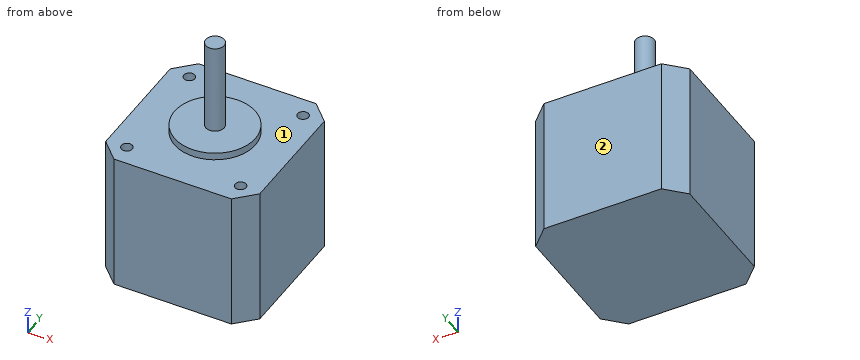
```python
from build123d import *

# Parameters (mm, degrees)
F0_W     = 42
F0_H     = 42
F1_DEPTH = 38
F2_SIZE  = 5
F3_R     = 11
F4_DEPTH = 2
F5_R     = 2.5
F6_DEPTH = 25
F7_R     = 1.5
F8_DEPTH = 25


with BuildPart() as f1:
    # F0 (on Top) → F1 (new body)
    with BuildSketch(Plane.XY):
        with Locations((21, 21)):
            Rectangle(F0_W, F0_H)
    extrude(amount=F1_DEPTH)

    # F2
    f2_edges = [f1.edges().sort_by_distance(p)[0] for p in [
        (0, 0, 19),
        (0, 42, 19),
        (42, 0, 19),
        (42, 42, 19),
    ]]
    chamfer(f2_edges, length=F2_SIZE)

    # F3 (on face) → F4 (join)
    with BuildSketch(Plane.XY.offset(38)):
        with Locations((21, 21)):
            Circle(F3_R)
    extrude(amount=F4_DEPTH)

    # F5 (on face) → F6 (join)
    with BuildSketch(Plane.XY.offset(40)):
        with Locations((21, 21)):
            Circle(F5_R)
    extrude(amount=F6_DEPTH)

    # F7 (on face) → F8 (cut)
    with BuildSketch(Plane.XY.offset(38)):
        with Locations((5.5, 36.5)):
            Circle(F7_R)
        with Locations((5.5, 5.5)):
            Circle(F7_R)
        with Locations((36.5, 36.5)):
            Circle(F7_R)
        with Locations((36.5, 5.5)):
            Circle(F7_R)
    extrude(amount=-F8_DEPTH, mode=Mode.SUBTRACT)


solid = f1.part
```
Geometry check sheet. Reference: the model listing, model coordinates, mm. Face numbers are marked on the shaded views. A direction names the side the tool comes from. Round coordinates to 2 decimals unless told otherwise and drop trailing zeros. Order: outer loops, then holes, each group sorted by start corner. A loop starts at its lowest first (then second) coordinate and runs counter-clockwise, first axis right, second up. Notation, with made-up numbers: (35.25, -36) - (84.25, -36) arc R20 ccw to (84.25, -10) - close; hole circle Ø7 at (44, 67). An arc over 180 degrees is marked (long way). Use a Markdown table: item, result. Add a question column.
1) Thickness scan on line 1 along Y through (x, z) = (36.5, 24); line 2 along X through (y, z) = (5, 26); line 3 along Z through (x, y) = (30, 32). Record the ranges inside material, lowest first.
2) Section check C-C (z = 26.5). Record the cut outline in (x, y).
3) Gauge pin test, flat ends, axial feed: P1, Ø12.5, axis at x = 18, y = 19.5, coming from the +Z side; P2, Ø0.9, axis at x = 36.5, y = 36, coming from the +Z side; P3, Ø12, axis at y = 10, z = 53.5, coming from the -X side; P4, Ø3.5, axis at x = 36.5, y = 36.5, coming from the +Z side. Record the tip position at first contact, or that the pin passes through.
4) Section check A-A (z = 11.5). Record the cut outline in (x, y).
5) Section check D-D (x = 16.5). Record the cut outline in (y, z), then the cut area to 3 significant figures.
6) Set-up check for the marked faces 1 and 2: record each of +Z, -Z, +X, -X, +Y, -Y from which the full face is reachable in a straight line by a thin tool's end or side.
7) Section check B-B (y = 21). Record the cut outline in (x, z), then the cut area to 4 significant figures.
Established:
| question | item | result |
|---|---|---|
| 1 | line 1 | 0 to 4, 7 to 35, 38 to 42 |
| 1 | line 2 | 0 to 4.09, 6.91 to 35.09, 37.91 to 42 |
| 1 | line 3 | 0 to 38 |
| 2 | outline | (0, 5) - (5, 0) - (37, 0) - (42, 5) - (42, 37) - (37, 42) - (5, 42) - (0, 37) - close; hole circle Ø3 at (5.5, 5.5); hole circle Ø3 at (5.5, 36.5); hole circle Ø3 at (36.5, 5.5); hole circle Ø3 at (36.5, 36.5) |
| 3 | P1 | z = 65 |
| 3 | P2 | z = 13 |
| 3 | P3 | through |
| 3 | P4 | z = 38 |
| 4 | outline | (0, 5) - (5, 0) - (37, 0) - (42, 5) - (42, 37) - (37, 42) - (5, 42) - (0, 37) - close |
| 5 | outline | (0, 0) - (42, 0) - (42, 38) - (31.04, 38) - (31.04, 40) - (10.96, 40) - (10.96, 38) - (0, 38) - close |
| 5 | area | 1,640 mm2 |
| 6 | face 1 | +Z |
| 6 | face 2 | +Z, -Z, +X, -X, +Y |
| 7 | outline | (0, 0) - (42, 0) - (42, 38) - (32, 38) - (32, 40) - (23.5, 40) - (23.5, 65) - (18.5, 65) - (18.5, 40) - (10, 40) - (10, 38) - (0, 38) - close |
| 7 | area | 1,765 mm2 |
